The figure shows three views and two pictorial views of one solid part (mm, origin at its lowest corner). Answer the questions. Coordinates: 2 decimals unless noted, no trailing zeros. Order: outer loops, then holes, each group sorted by start corner. A loop starts at its lowest first (then second) coordinate and runs counter-clockwise, first axis right, second up.
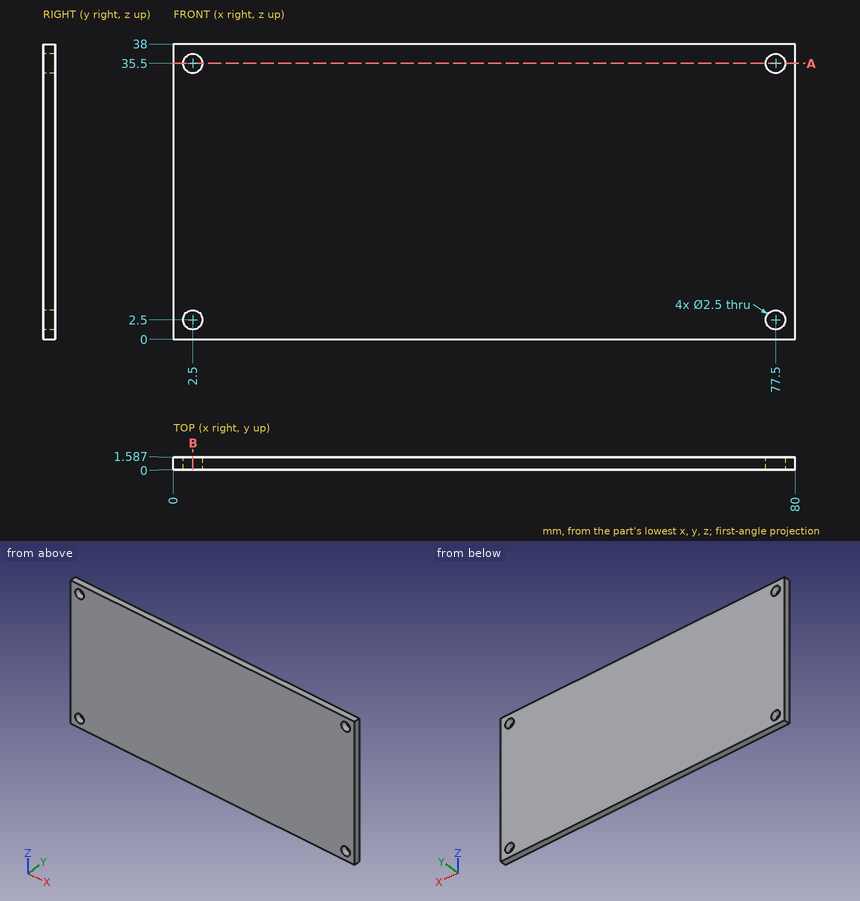
1) Each of these flat-tipped pins is pushed along its axis until it touches: P1, Ø2, axis at x = 77.5, z = 35.5, coming from the +Y side; P2, Ø3, axis at x = 2.5, z = 2.5, coming from the +Y side. Where does it stop, or does it pass through?
2) Straight lines are drawn through the part: probe 1 along Z at (x, y) = (2.5, 1.1); probe 2 along X at (y, z) = (1.45, 36.5). For each, find the intervals that lie inside material, in ascending order.
3) A cutting plane is placed at A-A, the plane z = 35.5. Write down the section's boundary in (x, y).
4) A cutting plane is placed at B-B, the plane x = 2.5. Write down the section's boundary in (y, z).
Working result:
1. P1: passes through
1. P2: stops at y = 1.59
2. probe 1: z = 0 to 1.25, 3.75 to 34.25, 36.75 to 38
2. probe 2: x = 0 to 1.75, 3.25 to 76.75, 78.25 to 80
3. outline: (0, 0) - (1.25, 0) - (1.25, 1.59) - (0, 1.59) - close; (3.75, 0) - (76.25, 0) - (76.25, 1.59) - (3.75, 1.59) - close; (78.75, 0) - (80, 0) - (80, 1.59) - (78.75, 1.59) - close
4. outline: (0, 0) - (1.59, 0) - (1.59, 1.25) - (0, 1.25) - close; (0, 3.75) - (1.59, 3.75) - (1.59, 34.25) - (0, 34.25) - close; (0, 36.75) - (1.59, 36.75) - (1.59, 38) - (0, 38) - close
